Part print with two shaded views. Sizes in mm from the minimum x, y, z corner. Round coordinates to 2 decimals unless told otherwise and drop trailing zeros. Write each loop counter-clockwise with the first axis right and the second up, starting at its lowest first coordinate (ties: lowest second). Pieces come first, ordered by that corner, then holes. Notation, with made-up numbers: (16, 69.25) -> (23, 69.25) arc R29 ccw to (23, 89.25) -> close; hole circle Ø10 at (25.5, 44.25). An arc over 180 degrees is marked (long way). Return JSON: item names as keys, results as strings. Group by question number.
(1) Saw through at A-A (x = 25). List the corners of the cut face in (y, z), plus the area to 3 significant figures.
(2) Saw through at D-D (y = 7.5). List the corners of the cut face in (x, z), plus the area to 3 significant figures.
(3) Drop flat-ended pins along their axis: pin 1 Ø2.5 at (x, z) = (25, 5.523) entering from +Y; pin 2 Ø2 at (x, z) = (18.5, 32) entering from -Y; pin 3 Ø1 at (x, y) = (14.5, 2) entering from -Z; pin 4 Ø1.5 at (x, z) = (15.5, 39) entering from -Y. Give the stop position or say it passes through.
(4) Saw through at B-B (z = 32). List the corners of the cut face in (x, y), plus the area to 3 significant figures.
(5) Saw through at C-C (x = 9.5). List the corners of the cut face in (y, z).
(6) Drill centre lines: L1, parallel to Z at x = 25, y = 5.45; L2, parallel to X at y = 4, z = 32; L3, parallel to Z at x = 15, y = 4.45. Where is each one in solid material? Low to high. Write a range as from..to.
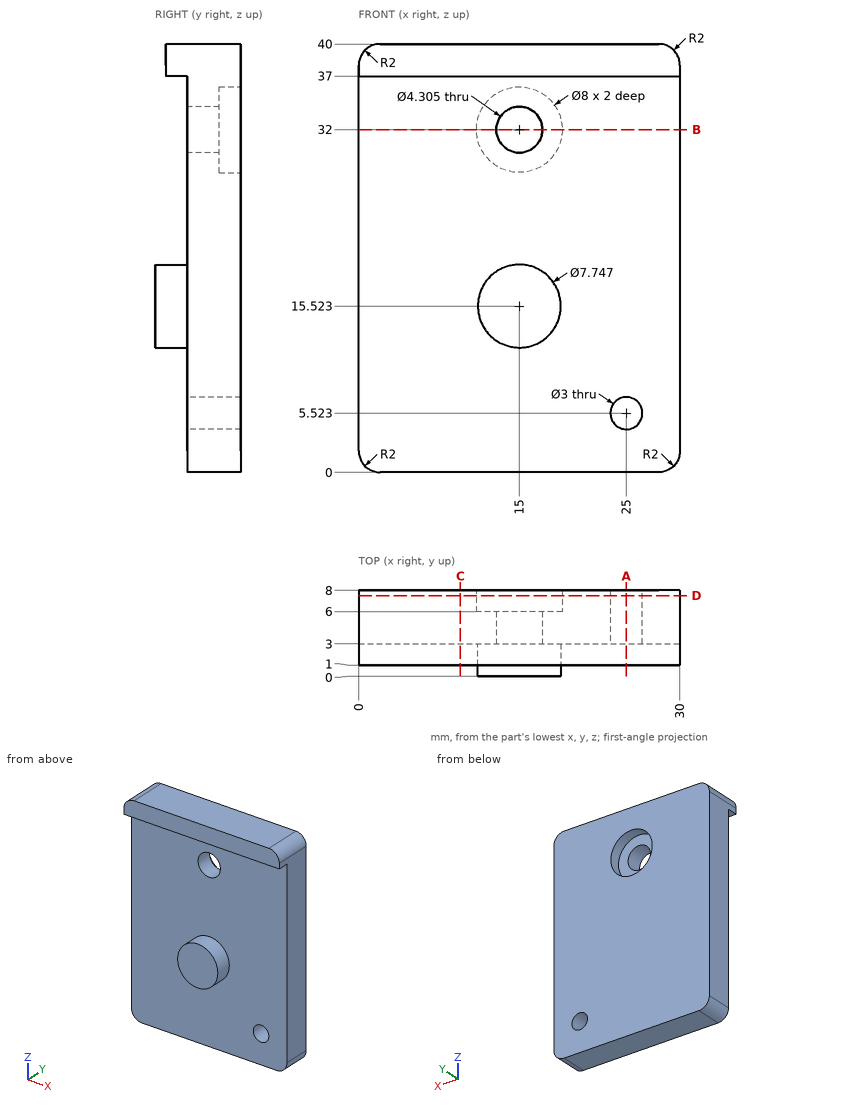
Computed values:
{
 "1": {"outline": "(1, 37) -> (3, 37) -> (3, 7.02) -> (8, 7.02) -> (8, 40) -> (1, 40) -> close; (3, 0) -> (8, 0) -> (8, 4.02) -> (3, 4.02) -> close", "area": "191 mm2"},
 "2": {"outline": "(0, 2) arc R2 ccw to (2, 0) -> (28, 0) arc R2 ccw to (30, 2) -> (30, 38) arc R2 ccw to (28, 40) -> (2, 40) arc R2 ccw to (0, 38) -> close; hole circle Ø8 at (15, 32); hole circle Ø3 at (25, 5.52)", "area": "1,140 mm2"},
 "3": {"pin 1": "through", "pin 2": "y = 3", "pin 3": "z = 11.65", "pin 4": "y = 1"},
 "4": {"outline": "(0, 3) -> (12.85, 3) -> (12.85, 6) -> (11, 6) -> (11, 8) -> (0, 8) -> close; (17.15, 3) -> (30, 3) -> (30, 8) -> (19, 8) -> (19, 6) -> (17.15, 6) -> close", "area": "121 mm2"},
 "5": {"outline": "(1, 37) -> (3, 37) -> (3, 0) -> (8, 0) -> (8, 40) -> (1, 40) -> close"},
 "6": {"L1": "0..4.02, 7.02..40", "L2": "0..12.85, 17.15..30", "L3": "0..29.85, 34.15..40"}
}
